Work out the finished part from the listing and answer in its coordinate system (mm). Face numbers are marked on the shaded views. Coordinates: 2 decimals unless noted, no trailing zeros. Loops run counter-clockwise (first coordinate to the right, second up) from the corner with the lowest first, then second, coordinate; pieces in that order, holes last. Notation, with made-up numbers: (26.5, 54) -> (73.5, 54) arc R7 ccw to (73.5, 62) -> close; hole circle Ø7 at (19.25, 7). An arc over 180 degrees is marked (long way). One line per question, with ' | ' between items.
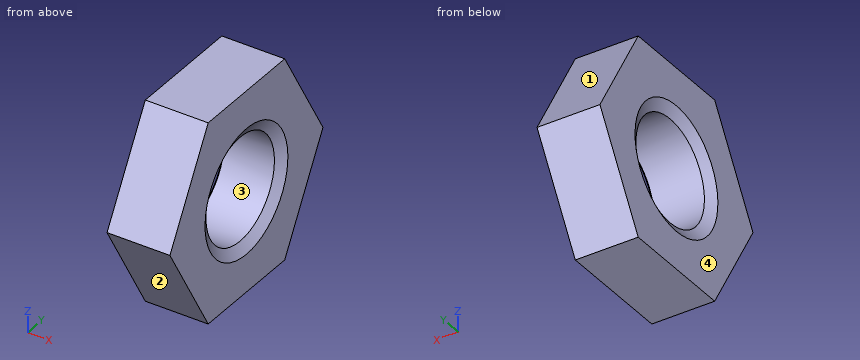
Autodesk Inventor part; units mm, degrees
ref_plane "Work Plane1" through (-9.9733, 0, 0) normal (0, 0, -1) x (1, 0, 0)
ref_plane "YZ Plane" through (0, 0, 0) normal (1, 0, 0) x (0, 1, 0)
ref_plane "XZ Plane" through (0, 0, 0) normal (0, 1, 0) x (-1, 0, 0)
sketch "Boceto1" plane through (0, 0, 0) normal (1, 0, 0) x (0, 1, 0)
  line L0 (2.3094, -4) -> (-2.3094, -4)
  line L1 (-2.3094, -4) -> (-4.6188, 0)
  line L2 (-4.6188, 0) -> (-2.3094, 4)
  line L3 (-2.3094, 4) -> (2.3094, 4)
  line L4 (2.3094, 4) -> (4.6188, 0)
  line L5 (4.6188, 0) -> (2.3094, -4)
  point P0 (0, 0)
  point P1 (0, 0)
  dimension "d0" = 9.2376
extrude "Cuerpo" add sketch "Boceto1" along normal blind 2.5
sketch "Boceto2" plane through (2.5, 0, 0) normal (1, 0, 0) x (0, 0, -1)
  point P0 (0, 0)
hole "Rosca" at (2.5, 0, 0) direction (-1, 0, 0) diameter 4.134 end through all
chamfer "Chaflán2" distance 0.433 angle 30 1 edges at (2.5, 0, 2.067) measured on face at (2.5, 2.8764, -1.7247)
chamfer "Chaflán1" distance 0.433 angle 30 1 edges at (0, 0, 2.067) measured on face at (0, 2.8764, -1.7247)
ref_plane "Work Plane1" through (-9.9733, 0, 0) normal (0, 0, -1) x (1, 0, 0)
equation "\"d0\" = 1.1547 * SW"
equation "\"d1\" = KOH"
equation "\"d12\" = -0.5 * GD1 + 0.5 * NND"
equation "\"d19\" = -0.5 * GD1 + 0.5 * NND"
equation "\"d10\" = -0.5 * GD1 + 0.5 * NND"
equation "\"d18\" = -0.5 * GD1 + 0.5 * NND"
equation "\"NND\" = 5"
equation "\"KOH\" = 2.5"
equation "\"SW\" = 8"
equation "\"GUL\" = 0.541266 * PTC"
equation "\"THREADDIA\" = 5"
equation "\"TOA\" = 30deg"
equation "\"PTC\" = 0.8"
equation "\"E0\" = 1.155 * SW"
equation "\"GAL\" = 0.541266 * PTC"
properties part number "BS 4183 - M5" material "Acero, suave"
1) Find section A-A (y = 0). Write down the section's boundary in (x, z), plus the area to 3 significant figures.
Check values:
outline: (0, -4) -> (2.5, -4) -> (2.5, -2.5) -> (2.25, -2.07) -> (0.25, -2.07) -> (0, -2.5) -> close; (0, 2.5) -> (0.25, 2.07) -> (2.25, 2.07) -> (2.5, 2.5) -> (2.5, 4) -> (0, 4) -> close | area: 9.45 mm^2
2) The mould has two halves that part along Z. Classify the marked faces 1, 2, 3 and 4: released by +Z, released by -Z, zero draft, split by the parting line, or undercut.
Check values:
face 1: released by +Z | face 2: released by -Z | face 3: undercut | face 4: zero draft
3) Find section C-C (y = 3). Write down the section's boundary in (x, z), plus the area to 3 significant figures.
Check values:
outline: (0, -2.8) -> (2.5, -2.8) -> (2.5, 2.8) -> (0, 2.8) -> close | area: 14.0 mm^2
4) Find the intervals of material crossed by line 1 along Z through (x, y) = (1.3, 0); line 2 along Z through (x, y) = (2.35, 0); line 3 along X through (y, z) = (-1.25, -2), in increasing order.
Check values:
line 1: z = -4 to -2.07, 2.07 to 4 | line 2: z = -4 to -2.24, 2.24 to 4 | line 3: x = 0.08 to 2.42
5) Find section B-B (x = 1.5). Write down the section's boundary in (y, z), plus the area to 3 significant figures.
Check values:
outline: (-4.62, 0) -> (-2.31, -4) -> (2.31, -4) -> (4.62, 0) -> (2.31, 4) -> (-2.31, 4) -> close; hole circle Ø4.13 at (0, 0) | area: 42.0 mm^2
